```python
from build123d import *

# Parameters (mm, degrees)
SKETCH2_W           = 30
SKETCH2_H           = 30
SKETCH2_R           = 14.5
BOSS_EXTRUDE1_DEPTH = 10.5
SKETCH3_R           = 8
BOSS_EXTRUDE2_DEPTH = 1
SKETCH4_R           = 1.5
CUT_EXTRUDE1_DEPTH  = 24.669600757
CUT_EXTRUDE2_DEPTH  = 7.5
FILLET1_R           = 0.5


with BuildPart() as part:
    # Sketch2 → Boss-Extrude1 (new body)
    with BuildSketch(Plane(origin=(0, 0, 0), x_dir=(1, 0, 0), z_dir=(0, 1, 0))):
        Rectangle(SKETCH2_W, SKETCH2_H)
        with Locations(Location((0, 0, 0), (0, 0, 90))):
            Circle(SKETCH2_R, mode=Mode.SUBTRACT)
    extrude(amount=BOSS_EXTRUDE1_DEPTH)

    # Sketch3 → Boss-Extrude2 (add)
    with BuildSketch(Plane.XZ):
        with BuildLine():
            Line((-1.15, 14.454324612), (-1.15, 11.25))
            Line((-1.15, 11.25), (-1.15, 7.916912277))
            ThreePointArc((-1.15, 7.916912277), (0, 8), (1.15, 7.916912277))
            Line((1.15, 7.916912277), (1.15, 11.25))
            Line((1.15, 11.25), (1.15, 14.454324612))
            ThreePointArc((1.15, 14.454324612), (0, 14.5), (-1.15, 14.454324612))
        make_face()
        Circle(SKETCH3_R)
        with BuildLine():
            ThreePointArc((11.942812309, -8.223091521), (12.557368355, -7.25), (13.092812309, -6.231233092))
            Line((13.092812309, -6.231233092), (10.317785793, -4.629070786))
            Line((10.317785793, -4.629070786), (7.431247151, -2.962526924))
            ThreePointArc((7.431247151, -2.962526924), (6.92820323, -4), (6.281247151, -4.954385353))
            Line((6.281247151, -4.954385353), (9.167785793, -6.620929214))
            Line((9.167785793, -6.620929214), (11.942812309, -8.223091521))
        make_face()
        with BuildLine():
            Line((-10.317785793, -4.629070786), (-13.092812309, -6.231233092))
            ThreePointArc((-13.092812309, -6.231233092), (-12.557368355, -7.25), (-11.942812309, -8.223091521))
            Line((-11.942812309, -8.223091521), (-9.167785793, -6.620929214))
            Line((-9.167785793, -6.620929214), (-6.281247151, -4.954385353))
            ThreePointArc((-6.281247151, -4.954385353), (-6.92820323, -4), (-7.431247151, -2.962526924))
            Line((-7.431247151, -2.962526924), (-10.317785793, -4.629070786))
        make_face()
    extrude(amount=-BOSS_EXTRUDE2_DEPTH)

    # Sketch4 → Cut-Extrude1 (cut, through all)
    with BuildSketch(Plane(origin=(0, 10.5, 0), x_dir=(1, 0, 0), z_dir=(0, 1, 0))):
        with BuildLine():
            Line((-15, 15), (-15, 11.936859783))
            ThreePointArc((-15, 11.936859783), (-14.102826997, 14.102826999), (-11.936859779, 15))
            Line((-11.936859779, 15), (-15, 15))
        make_face()
        with BuildLine():
            Line((15, 15), (11.936859768, 15))
            ThreePointArc((11.936859768, 15), (14.102826999, 14.102826997), (15, 11.936859766))
            Line((15, 11.936859766), (15, 15))
        make_face()
        with BuildLine():
            ThreePointArc((-11.936859768, -15), (-14.102826997, -14.102826998), (-15, -11.93685977))
            Line((-15, -11.93685977), (-15, -15))
            Line((-15, -15), (-11.936859768, -15))
        make_face()
        with BuildLine():
            ThreePointArc((15, -11.936859768), (14.102826999, -14.102826997), (11.93685977, -15))
            Line((11.93685977, -15), (15, -15))
            Line((15, -15), (15, -11.936859768))
        make_face()
        with Locations(Location((-12.02081528, 12.02081528, 0), (0, 0, 270))):
            Circle(SKETCH4_R)
        with Locations(Location((-12.02081528, -12.02081528, 0), (0, 0, 270))):
            Circle(SKETCH4_R)
        with Locations(Location((12.02081528, 12.02081528, 0), (0, 0, 270))):
            Circle(SKETCH4_R)
        with Locations(Location((12.02081528, -12.02081528, 0), (0, 0, 270))):
            Circle(SKETCH4_R)
    extrude(amount=-CUT_EXTRUDE1_DEPTH, mode=Mode.SUBTRACT)

    # Sketch4_3 → Cut-Extrude2 (cut)
    with BuildSketch(Plane(origin=(0, 10.5, 0), x_dir=(1, 0, 0), z_dir=(0, 1, 0))):
        with BuildLine():
            Line((-6.170782872, 15), (-11.936859779, 15))
            ThreePointArc((-11.936859779, 15), (-11.058003907, 14.871214971), (-10.253048327, 14.495689014))
            Line((-10.253048327, 14.495689014), (-9.899494937, 14.142135624))
            Line((-9.899494937, 14.142135624), (-8.263434371, 12.506075058))
            Line((-8.263434371, 12.506075058), (-6.170782872, 15))
        make_face()
        with BuildLine():
            Line((-12.506075058, 8.263434371), (-14.142135624, 9.899494937))
            Line((-14.142135624, 9.899494937), (-14.495689014, 10.253048327))
            ThreePointArc((-14.495689014, 10.253048327), (-14.871214971, 11.058003908), (-15, 11.936859783))
            Line((-15, 11.936859783), (-15, 6.170782872))
            Line((-15, 6.170782872), (-12.506075058, 8.263434371))
        make_face()
        with BuildLine():
            Line((11.936859768, 15), (6.170782872, 15))
            Line((6.170782872, 15), (8.263434371, 12.506075058))
            Line((8.263434371, 12.506075058), (9.899494937, 14.142135624))
            Line((9.899494937, 14.142135624), (10.253048327, 14.495689014))
            ThreePointArc((10.253048327, 14.495689014), (11.058003901, 14.871214969), (11.936859768, 15))
        make_face()
        with BuildLine():
            Line((14.142135624, 9.899494937), (12.506075058, 8.263434371))
            Line((12.506075058, 8.263434371), (15, 6.170782872))
            Line((15, 6.170782872), (15, 11.936859766))
            ThreePointArc((15, 11.936859766), (14.871214969, 11.0580039), (14.495689014, 10.253048327))
            Line((14.495689014, 10.253048327), (14.142135624, 9.899494937))
        make_face()
        with BuildLine():
            ThreePointArc((-10.253048327, -14.495689014), (-11.058003901, -14.871214969), (-11.936859768, -15))
            Line((-11.936859768, -15), (-6.170782872, -15))
            Line((-6.170782872, -15), (-8.263434371, -12.506075058))
            Line((-8.263434371, -12.506075058), (-9.899494937, -14.142135624))
            Line((-9.899494937, -14.142135624), (-10.253048327, -14.495689014))
        make_face()
        with BuildLine():
            Line((-12.506075058, -8.263434371), (-15, -6.170782872))
            Line((-15, -6.170782872), (-15, -11.93685977))
            ThreePointArc((-15, -11.93685977), (-14.871214969, -11.058003902), (-14.495689014, -10.253048327))
            Line((-14.495689014, -10.253048327), (-14.142135624, -9.899494937))
            Line((-14.142135624, -9.899494937), (-12.506075058, -8.263434371))
        make_face()
        with BuildLine():
            Line((15, -6.170782872), (12.506075058, -8.263434371))
            Line((12.506075058, -8.263434371), (14.142135624, -9.899494937))
            Line((14.142135624, -9.899494937), (14.495689014, -10.253048327))
            ThreePointArc((14.495689014, -10.253048327), (14.871214969, -11.058003901), (15, -11.936859768))
            Line((15, -11.936859768), (15, -6.170782872))
        make_face()
        with BuildLine():
            Line((9.899494937, -14.142135624), (8.263434371, -12.506075058))
            Line((8.263434371, -12.506075058), (6.170782872, -15))
            Line((6.170782872, -15), (11.93685977, -15))
            ThreePointArc((11.93685977, -15), (11.058003902, -14.871214969), (10.253048327, -14.495689014))
            Line((10.253048327, -14.495689014), (9.899494937, -14.142135624))
        make_face()
    extrude(amount=-CUT_EXTRUDE2_DEPTH, mode=Mode.SUBTRACT)

    # Fillet1
    fillet1_edges = [part.edges().sort_by_distance(p)[0] for p in [
        (-8.263434371, 6.75, 12.506075058),
        (-6.170782872, 6.75, 15),
        (15, 6.75, -6.170782872),
        (12.506075058, 6.75, -8.263434371),
        (8.263434371, 6.75, -12.506075058),
        (6.170782872, 6.75, -15),
        (-12.506075058, 6.75, -8.263434371),
        (-15, 6.75, -6.170782872),
        (-15, 6.75, 6.170782872),
        (-12.506075058, 6.75, 8.263434371),
        (12.506075058, 6.75, 8.263434371),
        (15, 6.75, 6.170782872),
        (6.170782872, 6.75, 15),
        (8.263434371, 6.75, 12.506075058),
        (-6.170782872, 6.75, -15),
        (-8.263434371, 6.75, -12.506075058),
    ]]
    fillet(fillet1_edges, radius=FILLET1_R)


solid = part.part
```
Check sheet for the modelled part. Datum: model origin and axes. Units: mm. A direction names the side the tool comes from. Coordinates: 2 decimals unless noted, no trailing zeros. Order: outer loops, then holes, each group sorted by start corner. A loop starts at its lowest first (then second) coordinate and runs counter-clockwise, first axis right, second up. Notation, with made-up numbers: M 2.25,-30.5 L 58.25,-30.5 A23 ccw 58.25,3.5 Z; hole C 71.25,57.25 d1. An arc over 180 degrees is marked long. Write each question's results on one line, items separated by ' | '. Start each with the question number.
1. Go/stop test with flat-tipped pins: P1, Ø2.5, axis at x = 12.02, z = -12.02, coming from the -Y side; P2, Ø11.5, axis at x = 6, z = 5.5, coming from the +Y side; P3, Ø0.5, axis at y = 0.5, z = 12.5, coming from the +X side; P4, Ø0.7, axis at x = -8.5, z = -13.5, coming from the +Y side. Record where each tip stops, or that it passes through.
2. Cross-section at C-C on z = -11.25. Record the cut outline in (x, y).
3. Cross-section at D-D on y = 2. Record the cut outline in (x, z), and give its area (3 significant figures).
4. Mould release check, pull along X, two halves, no side actions. Record for faces 1 (the face through (-13.68, 6.8, -9.44)), 2 (the face through (-1.15, 0.5, 11.2)), 3 (the face through (13.68, 6.8, 9.44)): +X half, -X half, draft (parallel to the pull), parting line (faces both ways), or undercut.
5. Cross-section at B-B on x = 0. Record the cut outline in (y, z).
6. Cross-section at A-A on z = 0. Record the cut outline in (x, y), and give its area (3 significant figures).
7. Material ranges on probe 1 along Z at (x, y) = (-0.5, 4.5); probe 2 along X at (y, z) = (4.75, 13); probe 3 along X at (y, z) = (7.25, -11), recorded low to high.
8. Access from +Z, -Z, +X, -X, +Y, -Y to the whole of each face (thin tool, end or side, straight path). Record for faces 4 (the face through (-0.1, 0.5, -8)), 5 (the face through (-13.886, 6.802, -7.106)), 6 (the face through (-9.462, 6.802, -13.705)), 7 (the face through (7.128, 6.802, 13.859)).
Checks:
1) P1: passes through | P2: stops at y = 1 | P3: stops at x = 14.98 | P4: stops at y = 3
2) outline: M -15,0 L -13.31,0 L -13.31,10.5 L -14.92,10.5 L -14.92,3 L -15,3 Z; M -10.73,0 L -9.15,0 L -9.15,10.5 L -10.73,10.5 Z; M 9.15,0 L 10.73,0 L 10.73,10.5 L 9.15,10.5 Z; M 13.31,0 L 15,0 L 15,3 L 14.92,3 L 14.92,10.5 L 13.31,10.5 Z
3) outline: M -15,-11.94 A3.06 ccw -11.94,-15 L 11.94,-15 A3.06 ccw 15,-11.94 L 15,11.94 A3.06 ccw 11.94,15 L -11.94,15 A3.06 ccw -15,11.94 Z; hole C 0,0 d29; hole C -12.02,-12.02 d3; hole C -12.02,12.02 d3; hole C 12.02,-12.02 d3; hole C 12.02,12.02 d3 | area: 203 mm²
4) face 1: -X half | face 2: undercut | face 3: +X half
5) outline: M 0,-15 L 10.5,-15 L 10.5,-14.5 L 0,-14.5 Z; M 0,-8 L 1,-8 L 1,14.5 L 10.5,14.5 L 10.5,15 L 0,15 Z
6) outline: M -15,0 L -14.5,0 L -14.5,10.5 L -15,10.5 Z; M -8,0 L 8,0 L 8,1 L -8,1 Z; M 14.5,0 L 15,0 L 15,10.5 L 14.5,10.5 Z | area: 26.5 mm²
7) probe 1: z = -15 to -14.49, 14.49 to 15 | probe 2: x = -14.81 to -13.16, -10.88 to -8.76, -7.85 to -6.42, 6.42 to 7.85, 8.76 to 10.88, 13.16 to 14.81 | probe 3: x = -14.85 to -13.12, -10.92 to -9.45, 9.45 to 10.92, 13.12 to 14.85
8) face 4: +Y, -Y | face 5: -X, +Y | face 6: -Z, +Y | face 7: +Z, +Y
